Verification items for the finished model (mm, model axes). Face numbers are marked on the shaded views. Give positions to 0.01 mm unless a question says otherwise; leave off trailing zeros. Order: outer loops, then holes, each group sorted by start corner. A loop starts at its lowest first (then second) coordinate and runs counter-clockwise, first axis right, second up. Notation, with made-up numbers: (66.25, 58.25) -> (81.25, 58.25) arc R27 cw to (81.25, 78.25) -> close; hole circle Ø4 at (-34, 85). An arc over 180 degrees is marked (long way). Write each question's results on one line, items separated by ' | '. Start each with the question number.
1. Cross-section at D-D, the plane z = 14. Enter the section's corners in (x, y), then the cut area to 3 significant figures.
2. Mould release check, pull along Z, two halves, no side actions. Record for the marked faces 1, 2 and 3: +Z half, -Z half, draft (parallel to the pull), parting line (faces both ways), or undercut.
3. Material ranges on L1, parallel to Y at x = 2, z = 40; L2, parallel to Z at x = 5, y = 2; L3, parallel to Y at x = 6, z = -27, recorded low to high. Write a range as from..to.
4. Cross-section at A-A, the plane y = 1. Enter the section's corners in (x, z).
5. Cross-section at C-C, the plane z = -28. Enter the section's corners in (x, y), then the cut area to 3 significant figures.
6. Cross-section at B-B, the plane y = -27. Enter the section's corners in (x, z).
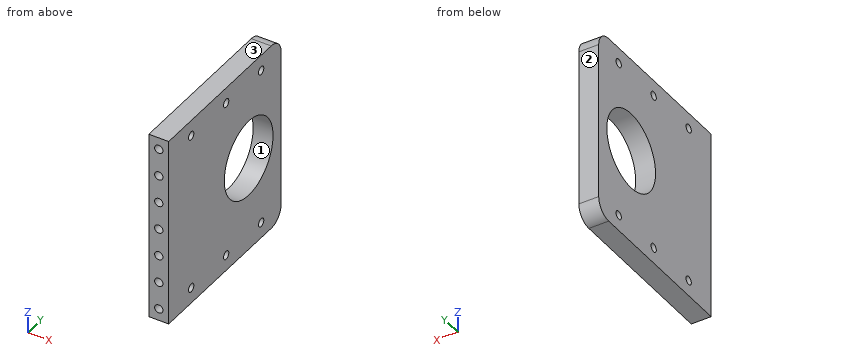
Autodesk Inventor part; units mm, degrees
ref_plane "YZ Plane" through (0, 0, 0) normal (1, 0, 0) x (0, 1, 0)
ref_plane "XZ Plane" through (0, 0, 0) normal (0, 1, 0) x (-1, 0, 0)
ref_plane "XY Plane" through (0, 0, 0) normal (0, 0, 1) x (1, 0, 0)
sketch "Sketch1" plane through (0, 0, 0) normal (1, 0, 0) x (0, 1, 0)
  line L0 (-45, 48) -> (45, 48)
  line L1 (45, 48) -> (45, -48)
  line L2 (45, -48) -> (-45, -48)
  line L3 (-45, -48) -> (-45, 48)
  line L4 (-45, 48) -> (45, -48) construction
  line L5 (45, 48) -> (-45, -48) construction
  point P0 (0, 0)
  dimension "d0" = 90
  dimension "d1" = 96
extrude "Extrusion1" add sketch "Sketch1" along normal blind 10
sketch "Sketch3" plane through (10, 0, 0) normal (1, 0, 0) x (0, 0, -1)
  circle A0 centre (0, 19) radius 19.5
  line L0 (-48, -45) -> (48, -45)
  point P0 (0, 0)
  point P1 (0, -45)
  dimension "d16" = 39
  dimension "d17" = 64
extrude "Extrusion3" cut sketch "Sketch3" against normal through all
sketch "Sketch5" plane through (10, 0, 0) normal (1, 0, 0) x (0, 0, -1)
  circle A0 centre (-40, 29) radius 2.1
  line L0 (-48, 45) -> (-48, -45) construction
  line L1 (-48, -45) -> (48, -45)
  circle A1 centre (-40, 1) radius 2.1
  circle A2 centre (-40, -27) radius 2.1
  circle A3 centre (0, 19) radius 19.5 construction
  line L2 (0, 38.5) -> (0, 19) construction
  circle A4 centre (40, 29) radius 2.1
  circle A5 centre (40, 1) radius 2.1
  circle A6 centre (40, -27) radius 2.1
  point P0 (0, 0)
  point P1 (-7.5, 41)
  point P2 (7.5, 41)
  dimension "d32" = 4.2
  dimension "d33" = 8
  dimension "d34" = 74
  dimension "d37" = 28
extrude "Extrusion5" cut sketch "Sketch5" against normal through all
sketch "Sketch6" plane through (0, -45, -48) normal (0, -1, 0) x (1, 0, 0)
  circle A0 centre (5, 90) radius 2.1
  line L0 (0, 96) -> (0, 0) construction
  line L1 (0, 96) -> (10, 96) construction
  circle A1 centre (5, 76) radius 2.1
  circle A2 centre (5, 62) radius 2.1
  circle A3 centre (5, 48) radius 2.1
  circle A4 centre (5, 34) radius 2.1
  circle A5 centre (5, 20) radius 2.1
  circle A6 centre (5, 6) radius 2.1
  point P0 (0, 48)
  point P1 (0, 48)
  point P2 (5, 96)
  dimension "d44" = 4.2
  dimension "d45" = 42
  dimension "d48" = 14
extrude "Extrusion6" cut sketch "Sketch6" against normal blind 10
thread "Thread1"
thread "Thread2"
thread "Thread3"
thread "Thread4"
thread "Thread5"
thread "Thread6"
thread "Thread7"
fillet "Fillet1" radius 8 2 edges at (5, 45, 48) (5, 45, -48)
properties part number "ArmSupportPlate" material "Aluminum 6061"
Results below:
1) outline: (0, -45) -> (2.9, -45) -> (2.9, -35) -> (7.1, -35) -> (7.1, -45) -> (10, -45) -> (10, 5.43) -> (0, 5.43) -> close; (0, 32.57) -> (10, 32.57) -> (10, 45) -> (0, 45) -> close | area: 587 mm²
2) face 1: undercut | face 2: draft | face 3: +Z half
3) L1: y = -45..-29.1, -24.9..-1.1, 3.1..26.9, 31.1..45 | L2: z = -48..-41.85, -38.15..-9.55, 9.55..38.15, 41.85..48 | L3: y = -35..45
4) outline: (0, -48) -> (10, -48) -> (10, -42.1) -> (0, -42.1) -> close; (0, -37.9) -> (10, -37.9) -> (10, -7.5) -> (0, -7.5) -> close; (0, 7.5) -> (10, 7.5) -> (10, 37.9) -> (0, 37.9) -> close; (0, 42.1) -> (10, 42.1) -> (10, 48) -> (0, 48) -> close
5) outline: (0, -45) -> (2.9, -45) -> (2.9, -35) -> (7.1, -35) -> (7.1, -45) -> (10, -45) -> (10, 45) -> (0, 45) -> close | area: 858 mm²
6) outline: (0, -48) -> (10, -48) -> (10, -42.1) -> (0, -42.1) -> close; (0, -37.9) -> (10, -37.9) -> (10, 37.9) -> (0, 37.9) -> close; (0, 42.1) -> (10, 42.1) -> (10, 48) -> (0, 48) -> close
